Study the drawing (mm; zero at the part's minimum x, y, z) and answer. Round coordinates to 2 decimals unless told otherwise and drop trailing zeros. Write each loop counter-clockwise with the first axis right and the second up, starting at its lowest first coordinate (ties: lowest second). Pieces come first, ordered by that corner, then holes.
(1) A cutting plane is placed at A-A, the plane x = 38.1. Give the vertices of the cut face in (y, z).
(2) Find the intervals of material crossed by probe 1 along Z at (x, y) = (9, 2.5); probe 2 along Z at (x, y) = (7.5, 2.75) (1 decimal); probe 3 along X at (y, z) = (1.25, 8) (1 decimal), in increasing order.
(3) This flat-tipped pin is pushed along its axis until it touches: pin 1 Ø4 at (x, z) = (67.22, 67.22) entering from -Y. Where does it stop, or does it pass through?
(4) A cutting plane is placed at B-B, the plane y = 4.75. Give the vertices of the cut face in (x, z) (1 decimal).
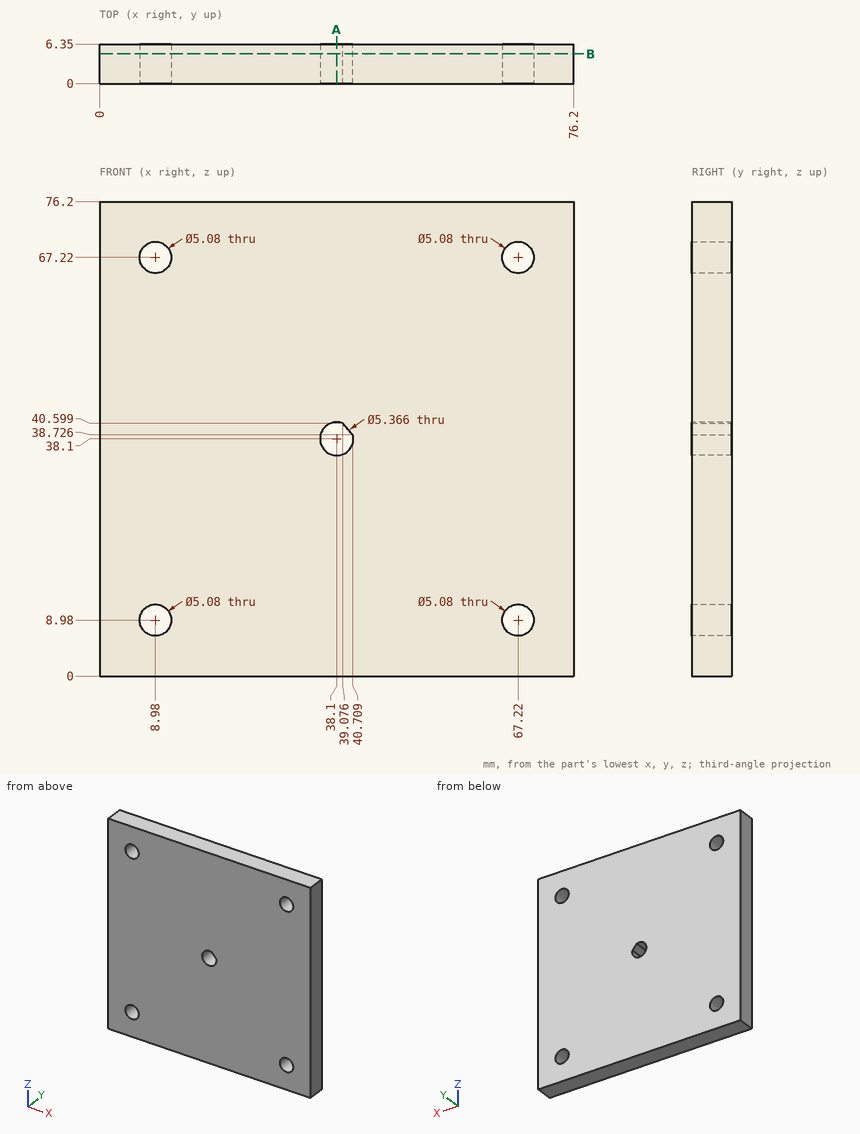
Solutions:
1. outline: (0, 0) - (6.35, 0) - (6.35, 35.42) - (0, 35.42) - close; (0, 40.78) - (6.35, 40.78) - (6.35, 76.2) - (0, 76.2) - close
2. probe 1: z = 0 to 6.44, 11.52 to 64.68, 69.76 to 76.2
2. probe 2: z = 0 to 6.9, 11 to 65.2, 69.3 to 76.2
2. probe 3: x = 0 to 6.6, 11.3 to 64.9, 69.6 to 76.2
3. pin 1: passes through
4. outline: (0, 0) - (76.2, 0) - (76.2, 76.2) - (0, 76.2) - close; hole circle Ø5.1 at (9, 9); hole circle Ø5.1 at (9, 67.2); hole (39.1, 40.6) arc R2.7 ccw (long way) to (40.7, 38.7) - close; hole circle Ø5.1 at (67.2, 9); hole circle Ø5.1 at (67.2, 67.2)
